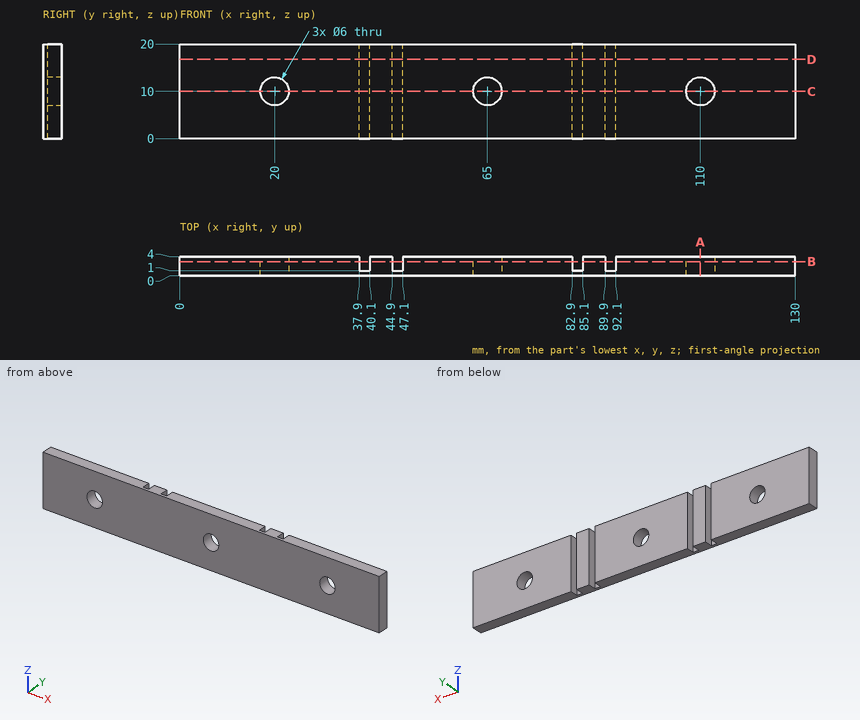
Study the drawing (mm; zero at the part's minimum x, y, z) and answer. Give positions to 0.01 mm unless a question says otherwise; leave off trailing zeros. Order: outer loops, then holes, each group sorted by start corner. A loop starts at its lowest first (then second) coordinate and runs counter-clockwise, first axis right, second up. Notation, with made-up numbers: (0.5, 41) -> (28.5, 41) arc R26 ccw to (28.5, 74) -> close; hole circle Ø9 at (6, 18). An arc over 180 degrees is marked (long way). Put each result on its own line as item: value.
Item 1: Given P1, Ø1.1, axis at x = 91, z = 6.5, coming from the +Y side, flat-ended and moving along its own axis, determine where the tip first touches the part or whether it passes through.
Established:
P1: stops at y = 1
Item 2: A cutting plane is placed at B-B on y = 2.95. Give the vertices of the cut face in (x, z), plus the area to 3 significant figures.
Established:
outline: (0, 0) -> (37.9, 0) -> (37.9, 20) -> (0, 20) -> close; (40.1, 0) -> (44.9, 0) -> (44.9, 20) -> (40.1, 20) -> close; (47.1, 0) -> (82.9, 0) -> (82.9, 20) -> (47.1, 20) -> close; (85.1, 0) -> (89.9, 0) -> (89.9, 20) -> (85.1, 20) -> close; (92.1, 0) -> (130, 0) -> (130, 20) -> (92.1, 20) -> close; hole circle Ø6 at (20, 10); hole circle Ø6 at (65, 10); hole circle Ø6 at (110, 10)
area: 2,340 mm^2
Item 3: Straight lines are drawn through the part: line 1 (X direction, y = 1.4, z = 14.75); line 2 (Z direction, x = 110, y = 1.35); line 3 (X direction, y = 0.6, z = 8.5). For each, find the intervals that lie inside material, in ascending order.
Established:
line 1: x = 0 to 37.9, 40.1 to 44.9, 47.1 to 82.9, 85.1 to 89.9, 92.1 to 130
line 2: z = 0 to 7, 13 to 20
line 3: x = 0 to 17.4, 22.6 to 62.4, 67.6 to 107.4, 112.6 to 130
Item 4: A cutting plane is placed at D-D on z = 16.75. Give the vertices of the cut face in (x, y).
Established:
outline: (0, 0) -> (130, 0) -> (130, 4) -> (92.1, 4) -> (92.1, 1) -> (89.9, 1) -> (89.9, 4) -> (85.1, 4) -> (85.1, 1) -> (82.9, 1) -> (82.9, 4) -> (47.1, 4) -> (47.1, 1) -> (44.9, 1) -> (44.9, 4) -> (40.1, 4) -> (40.1, 1) -> (37.9, 1) -> (37.9, 4) -> (0, 4) -> close
Item 5: A cutting plane is placed at C-C on z = 10. Count the separate pieces of the cut face and the enclosed holes in it, plus the area to 3 significant figures.
Established:
separate pieces: 4
enclosed holes: 0
area: 422 mm^2
Item 6: A cutting plane is placed at A-A on x = 110. Give the vertices of the cut face in (y, z).
Established:
outline: (0, 0) -> (4, 0) -> (4, 7) -> (0, 7) -> close; (0, 13) -> (4, 13) -> (4, 20) -> (0, 20) -> close
